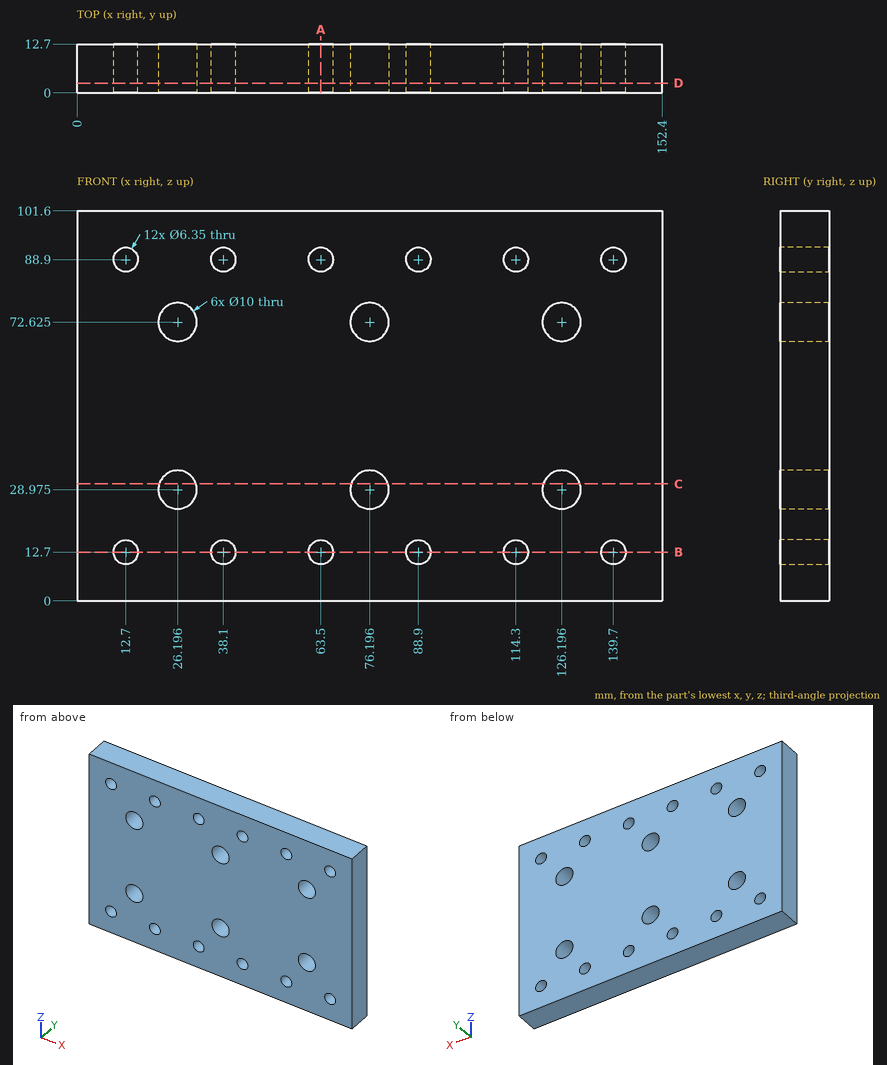
Source: three-view drawing plus pictorial views. Frame: mm from the lowest corner of the part. Coordinates: 2 decimals unless noted, no trailing zeros. Write each loop counter-clockwise with the first axis right and the second up, starting at its lowest first coordinate (ties: lowest second). Pieces come first, ordered by that corner, then holes. Notation, with made-up numbers: (65, 27.5) - (121, 27.5) arc R24 cw to (121, 37.5) - close; hole circle Ø10 at (-6.75, 39). An arc over 180 degrees is marked (long way). Answer as a JSON object with one key per item and string values.
Q1. Section query A-A, the plane x = 63.5. Output: boundary loops of the cut face in (y, z) (3 decimals), plus the area to 3 significant figures.
Ans:
{"outline": "(0, 0) - (12.7, 0) - (12.7, 9.525) - (0, 9.525) - close; (0, 15.875) - (12.7, 15.875) - (12.7, 85.725) - (0, 85.725) - close; (0, 92.075) - (12.7, 92.075) - (12.7, 101.6) - (0, 101.6) - close", "area": "1,130 mm2"}
Q2. First-contact query: pin 1 Ø5 at (x, y) = (102.5, 2) entering from -Z. Flat tip, straight axial feed; report the tip coordinate or a pass-through.
Ans:
{"pin 1": "stops at z = 0"}
Q3. Material intervals for line 1 (Z direction, x = 139.7, y = 4.25) (3 decimals); line 2 (Z direction, x = 122, y = 4) (1 decimal); line 3 (X direction, y = 6.5, z = 30.5), sorted ascending. Write a range as [from, to].
Ans:
{"line 1": "z = [0, 9.525], [15.875, 85.725], [92.075, 101.6]", "line 2": "z = [0, 26.3], [31.7, 69.9], [75.3, 101.6]", "line 3": "x = [0, 21.43], [30.96, 71.43], [80.96, 121.43], [130.96, 152.4]"}
Q4. Section query B-B, the plane z = 12.7. Output: boundary loops of the cut face in (x, y) (3 decimals).
Ans:
{"outline": "(0, 0) - (9.525, 0) - (9.525, 12.7) - (0, 12.7) - close; (15.875, 0) - (34.925, 0) - (34.925, 12.7) - (15.875, 12.7) - close; (41.275, 0) - (60.325, 0) - (60.325, 12.7) - (41.275, 12.7) - close; (66.675, 0) - (85.725, 0) - (85.725, 12.7) - (66.675, 12.7) - close; (92.075, 0) - (111.125, 0) - (111.125, 12.7) - (92.075, 12.7) - close; (117.475, 0) - (136.525, 0) - (136.525, 12.7) - (117.475, 12.7) - close; (142.875, 0) - (152.4, 0) - (152.4, 12.7) - (142.875, 12.7) - close"}
Q5. Section query C-C, the plane z = 30.5. Output: boundary loops of the cut face in (x, y), plus the area to 3 significant figures.
Ans:
{"outline": "(0, 0) - (21.43, 0) - (21.43, 12.7) - (0, 12.7) - close; (30.96, 0) - (71.43, 0) - (71.43, 12.7) - (30.96, 12.7) - close; (80.96, 0) - (121.43, 0) - (121.43, 12.7) - (80.96, 12.7) - close; (130.96, 0) - (152.4, 0) - (152.4, 12.7) - (130.96, 12.7) - close", "area": "1,570 mm2"}
Q6. Section query D-D, the plane y = 2.5. State how many separate pieces and enclosed holes the cut face has, plus the area to 3 significant figures.
Ans:
{"separate pieces": "1", "enclosed holes": "18", "area": "14,600 mm2"}
